from build123d import *

# Parameters (mm, degrees)
F0_R     = 1
F0_W     = 5
F0_H     = 3.2
F1_DEPTH = 4
F2_R     = 1.5
F3_R     = 1.5
F4_DEPTH = 5
F5_R     = 1.5


with BuildPart() as f1:
    # F0 (on Front) → F1 (new body)
    with BuildSketch(Plane.XZ):
        with BuildLine():
            Line((5, 3.1), (-3.5, 3.1))
            ThreePointArc((-3.5, 3.1), (-3.93934, 2.03934), (-5, 1.6))
            Line((-5, 1.6), (0, 1.6))
            Line((0, 1.6), (0, -1.6))
            Line((0, -1.6), (-5, -1.6))
            ThreePointArc((-5, -1.6), (-3.93934, -2.03934), (-3.5, -3.1))
            Line((-3.5, -3.1), (5, -3.1))
            Line((5, -3.1), (5, 3.1))
        make_face()
        with Locations((1.5, 0)):
            Circle(F0_R, mode=Mode.SUBTRACT)
        with Locations((-2.5, 0)):
            Rectangle(F0_W, F0_H)
    extrude(amount=F1_DEPTH)

    # F2
    f2_edges = [f1.edges().sort_by_distance(p)[0] for p in [
        (-3.5, -2, 3.1),
        (-3.5, -2, -3.1),
    ]]
    fillet(f2_edges, radius=F2_R)

    # F3 (on face) → F4 (cut)
    with BuildSketch(Plane(origin=(-5, 0, 0), x_dir=(0, -1, 0), z_dir=(-1, 0, 0))):
        with Locations((2, 0)):
            Circle(F3_R)
    extrude(amount=-F4_DEPTH, mode=Mode.SUBTRACT)

    # F5
    f5_edges = [f1.edges().sort_by_distance(p)[0] for p in [
        (5, -2, 3.1),
        (1.299038, -4, 3.1),
        (1.299038, 0, 3.1),
        (5, -2, -3.1),
        (1.299038, -4, -3.1),
        (1.299038, 0, -3.1),
    ]]
    fillet(f5_edges, radius=F5_R)


solid = f1.part
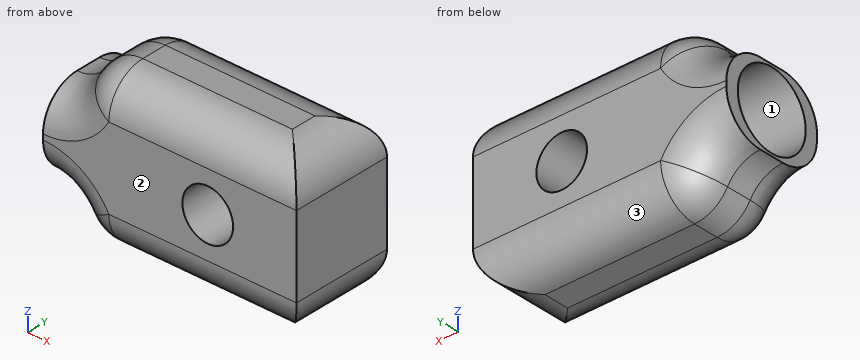
The model under review builds one solid part; all positions refer to its coordinate system, in mm. Face numbers are marked on the shaded views. Coordinates: 2 decimals unless noted, no trailing zeros. Write each loop counter-clockwise with the first axis right and the second up, starting at its lowest first coordinate (ties: lowest second). Pieces come first, ordered by that corner, then holes. Notation, with made-up numbers: (17, 40) - (38, 40) arc R23 ccw to (38, 58) - close; hole circle Ø2 at (-32.75, -30.75). An arc over 180 degrees is marked (long way). Answer as a JSON object with one key per item and string values. Group by question number.
1. Add section C-C (x = -1). Give the boundary of the cut face in (y, z).
2. Add section B-B (y = -2). Give the boundary of the cut face in (x, z).
3. Mouldability with a two-part tool opening along Y and no side actions: class the marked faces 1, 2 and 3 as pulls with the +Y half, pulls with the -Y half, needs draft (parallel to the pull), parting line crosses it, or undercut.
4. To check wall thickness, follow probe 1 along Z at (x, y) = (1.5, -2.45); probe 2 along X at (y, z) = (-1.5, 0.75); probe 3 along Z at (x, y) = (-1.7, -2). State the ranges of each line that lie inside material, in increasing order.
5. Clearance check with flat-ended pins moving along their axes: pin 1 Ø1.5 at (x, z) = (-3.5, 1) entering from -Y; pin 2 Ø1.8 at (x, z) = (1.5, 0) entering from -Y; pin 3 Ø1.5 at (y, z) = (-2.5, 0.5) entering from -X. State where each tip first meets the part, or that it passes through.
6. Add section A-A (z = 0). Give the boundary of the cut face in (x, y).
7. Add section D-D (x = 1.5). Give the boundary of the cut face in (y, z).
Findings:
{
 "1": {"outline": "(-4, -1.6) arc R1.5 ccw to (-2.5, -3.1) - (-1.5, -3.1) arc R1.5 ccw to (0, -1.6) - (0, 1.6) arc R1.5 ccw to (-1.5, 3.1) - (-2.5, 3.1) arc R1.5 ccw to (-4, 1.6) - close; hole circle Ø3 at (-2, 0)"},
 "2": {"outline": "(-5, -1.6) arc R1.5 cw to (-3.7, -2.35) arc R1.5 ccw to (-2.4, -3.1) - (3.5, -3.1) arc R1.5 ccw to (5, -1.6) - (5, 1.6) arc R1.5 ccw to (3.5, 3.1) - (-2.4, 3.1) arc R1.5 ccw to (-3.7, 2.35) arc R1.5 cw to (-5, 1.6) - (-5, 1.5) - (0, 1.5) - (0, -1.5) - (-5, -1.5) - close; hole circle Ø2 at (1.5, 0)"},
 "3": {"face 1": "undercut", "face 2": "pulls with the -Y half", "face 3": "pulls with the +Y half"},
 "4": {"probe 1": "-3.1 to -1, 1 to 3.1", "probe 2": "0 to 0.84, 2.16 to 5", "probe 3": "-3.1 to -1.5, 1.5 to 3.1"},
 "5": {"pin 1": "y = -4", "pin 2": "through", "pin 3": "x = 0"},
 "6": {"outline": "(-5, -4) - (0.5, -4) - (0.5, 0) - (-5, 0) - (-5, -0.5) - (0, -0.5) - (0, -3.5) - (-5, -3.5) - close; (2.5, -4) - (5, -4) - (5, 0) - (2.5, 0) - close"},
 "7": {"outline": "(-4, -1.6) arc R1.5 ccw to (-2.5, -3.1) - (-1.5, -3.1) arc R1.5 ccw to (0, -1.6) - (0, -1) - (-4, -1) - close; (-4, 1) - (0, 1) - (0, 1.6) arc R1.5 ccw to (-1.5, 3.1) - (-2.5, 3.1) arc R1.5 ccw to (-4, 1.6) - close"}
}
